```python
from build123d import *

# Parameters (mm, degrees)
EXTRUDE_17_DEPTH     = 2
SKETCH_4_R           = 3.35601343
CUT_EXTRUDE_25_DEPTH = 45.170960421


with BuildPart() as part:
    # 草图2 → 凸台-拉伸17 (new body)
    with BuildSketch(Plane(origin=(0, 0, 0), x_dir=(1, 0, 0), z_dir=(0, 1, 0))):
        with BuildLine():
            Line((-4.904700538, 30.145825623), (-28.559401011, -10.825317434))
            ThreePointArc((-28.559401011, -10.825317434), (-28.55940111, -16.488777843), (-23.654700538, -19.320508076))
            Line((-23.654700538, -19.320508076), (23.654700538, -19.320508076))
            ThreePointArc((23.654700538, -19.320508076), (28.559401192, -16.4887777), (28.559400847, -10.825317149))
            Line((28.559400847, -10.825317149), (4.904700538, 30.145825623))
            ThreePointArc((4.904700538, 30.145825623), (0, 32.977555799), (-4.904700538, 30.145825623))
        make_face()
        Polygon((-7.447524928, -4.330127019), (-13.79282439, -15.320508076), (-20.138123851, -4.330127019), align=None, mode=Mode.SUBTRACT)
        Polygon((5.190598923, -4.330127019), (12.690598923, -17.320508076), (-12.690598923, -17.320508076), (-5.190598923, -4.330127019), align=None, mode=Mode.SUBTRACT)
        Polygon((7.5, -4.330127019), (20.190598923, -4.330127019), (13.845299462, -15.320508076), align=None, mode=Mode.SUBTRACT)
        Polygon((-6.345299462, -2.330127019), (-21.345299462, -2.330127019), (-8.654700538, 19.650635095), (-1.154700538, 6.660254038), align=None, mode=Mode.SUBTRACT)
        Polygon((0, 8.660254038), (-6.345299462, 19.650635095), (6.345299462, 19.650635095), align=None, mode=Mode.SUBTRACT)
        Polygon((1.154700538, 6.660254038), (8.654700538, 19.650635095), (8.930688533, 19.172609866), (21.345299462, -2.330127019), (6.345299461, -2.330127019), align=None, mode=Mode.SUBTRACT)
    extrude(amount=EXTRUDE_17_DEPTH)

    # 草图4 → 切除-拉伸25 (cut, through all)
    with BuildSketch(Plane(origin=(0, 2, 0), x_dir=(1, 0, 0), z_dir=(0, 1, 0))):
        with Locations(Location((0, 0, 0), (0, 0, 270))):
            Circle(SKETCH_4_R)
    extrude(amount=-CUT_EXTRUDE_25_DEPTH, mode=Mode.SUBTRACT)


solid = part.part
```
For this review, take the finished solid that the model builds, in its own axes (mm). A direction names the side the tool comes from. Coordinates: 2 decimals unless noted, no trailing zeros. Order: outer loops, then holes, each group sorted by start corner. A loop starts at its lowest first (then second) coordinate and runs counter-clockwise, first axis right, second up. Notation, with made-up numbers: (12, 9) - (34, 9) arc R11 cw to (34, 29) - close; hole circle Ø10 at (13.25, 80.5). An arc over 180 degrees is marked (long way). Answer as a JSON object with one key per item and string values. Group by question number.
1. We need section D-D on z = 10. State the section outline as (x, y) points.
2. We need section B-B on z = -12. State the section outline as (x, y) points.
3. For probe 1 along Z at (x, y) = (20, 0.8); probe 2 along X at (y, z) = (0.75, 0); probe 3 along Z at (x, y) = (-1.5, 1.45), list the stretches that pass through material, from the lowest coordinate up.
4. We need section A-A on y = 1.2. State the section outline as (x, z) points.
5. The part is to be moulded in two halves that separate along X. For faces 3 (the flat face through (4, 0, 1)), 4 (the flat face through (16.9, 0.99, -9.37)), 5 (the flat face through (0, 1, -19.651)), say which applies: pulls with the +X half, pulls with the -X half, needs draft (parallel to the pull), parting line crosses it, or undercut.
6. For faces 1 (the flat face through (10.717, 0.986, 9.902)), 2 (the cylindrical face through (-28.6, 0.99, 16.42)), list the 3-axis set-ups (+Z, -Z, +X, -X, +Y, -Y) from which the entire face can be reached by the end or side of a thin tool; tool diameter is ignored.
7. Clearance check with flat-ended pins moving along their axes: P1, Ø0.6, axis at x = -11, y = 0.5, coming from the -Z side; P2, Ø1, axis at x = -14.5, y = 1, coming from the -Z side; P3, Ø6, axis at x = 0, z = 0, coming from the +Y side. State where each tip first meets the part, or that it passes through.
8. We need section C-C on z = -6. State the section outline as (x, y) points.
Final values:
{
 "1": {"outline": "(-28.08, 0) - (-16.86, 0) - (-16.86, 2) - (-28.08, 2) - close; (-10.72, 0) - (-8.46, 0) - (-8.46, 2) - (-10.72, 2) - close; (8.46, 0) - (10.77, 0) - (10.77, 2) - (8.46, 2) - close; (16.92, 0) - (28.08, 0) - (28.08, 2) - (16.92, 2) - close"},
 "2": {"outline": "(-15.38, 0) - (-13.07, 0) - (-13.07, 2) - (-15.38, 2) - close; (-4.24, 0) - (-1.93, 0) - (-1.93, 2) - (-4.24, 2) - close; (1.93, 0) - (4.24, 0) - (4.24, 2) - (1.93, 2) - close; (13.07, 0) - (15.38, 0) - (15.38, 2) - (13.07, 2) - close"},
 "3": {"probe 1": "-4 to 0, 2.33 to 4.33, 4.66 to 19.32", "probe 2": "-22.31 to -20, -5 to -3.36, 3.36 to 5, 20 to 22.31", "probe 3": "-32.78 to -19.65, -11.26 to -7.26, -6.06 to -3, 3 to 4.33, 17.32 to 19.32"},
 "4": {"outline": "(-28.56, 10.83) - (-4.9, -30.15) arc R5.66 ccw to (4.9, -30.15) - (28.56, 10.83) arc R5.66 ccw to (23.65, 19.32) - (-23.65, 19.32) arc R5.66 ccw to start; hole (-21.35, 2.33) - (-8.65, -19.65) - (-1.15, -6.66) - (-6.35, 2.33) - close; hole (-20.14, 4.33) - (-7.45, 4.33) - (-13.79, 15.32) - close; hole (-12.69, 17.32) - (-5.19, 4.33) - (5.19, 4.33) - (12.69, 17.32) - close; hole (-6.35, -19.65) - (6.35, -19.65) - (0, -8.66) - close; hole circle Ø6.71 at (0, 0); hole (1.15, -6.66) - (8.65, -19.65) - (21.35, 2.33) - (6.35, 2.33) - close; hole (7.5, 4.33) - (20.19, 4.33) - (13.85, 15.32) - close"},
 "5": {"face 3": "needs draft", "face 4": "pulls with the +X half", "face 5": "undercut"},
 "6": {"face 1": "+Y, -Y", "face 2": "-X, +Y, -Y"},
 "7": {"P1": "z = -20.11", "P2": "z = -14.39", "P3": "through"},
 "8": {"outline": "(-18.85, 0) - (-16.54, 0) - (-16.54, 2) - (-18.85, 2) - close; (-1.54, 0) - (1.54, 0) - (1.54, 2) - (-1.54, 2) - close; (16.54, 0) - (18.85, 0) - (18.85, 2) - (16.54, 2) - close"}
}
